```python
from build123d import *

# Parameters (mm, degrees)
F0_W        = 25
F0_H        = 25
F0_R        = 7.5
F1_DEPTH    = 35
F2_DEPTH    = 15
F3_SIZE2    = 21.650625
F3_SIZE     = 12.49999
F4_R        = 7.5
F5_DEPTH    = 5
F6_T1_DEPTH = 95.1228407313
F6_T3_DEPTH = 95.1228407313


# Not quite as in the source:
# - a fillet or chamfer that OpenCascade refuses, or shapes differently, is made with other operations: its cross-section is extruded or revolved along the edge and cut away or added
# - a fillet or chamfer is up to 0.001 mm smaller than in the source, because OpenCascade refuses the exact size


with BuildPart() as f1:
    # F0 (on Top) → F1 (new body)
    with BuildSketch(Plane.XY):
        with Locations((-12.5, -12.5)):
            Rectangle(F0_W, F0_H)
        with Locations((-12.5, -12.5)):
            Circle(F0_R, mode=Mode.SUBTRACT)
        with Locations((-12.5, -12.5)):
            Circle(F0_R)
    extrude(amount=F1_DEPTH)

    # F0 (on Top) → F2 (cut)
    with BuildSketch(Plane.XY):
        with Locations((-12.5, -12.5)):
            Circle(F0_R)
    extrude(amount=F2_DEPTH, mode=Mode.SUBTRACT)

    # F3 (size 12.5 and 21.6506350946 in the source; OpenCascade refuses exactly that, so slightly less here)
    f3_edges = [f1.edges().sort_by_distance(p)[0] for p in [
        (-25, -12.5, 35),
        (-12.5, -25, 35),
        (0, -12.5, 35),
        (-12.5, 0, 35),
    ]]
    f3_side = f1.faces().sort_by_distance((-12.5, -12.5, 35))[0]
    chamfer(f3_edges, length=F3_SIZE, length2=F3_SIZE2, reference=f3_side)

    # F4 (on Top) → F5 (join)
    with BuildSketch(Plane.XY):
        Polygon((-3.4594764784, -16.2579490188), (-3.4594764784, -8.802104896), (-8.731554417, -3.5300269574), (-16.1873985398, -3.5300269574), (-21.4594764784, -8.802104896), (-21.4594764784, -16.2579490188), (-16.1873985398, -21.5300269574), (-8.731554417, -21.5300269574), align=None)
        with Locations((-12.4594764784, -12.5300269574)):
            Circle(F4_R, mode=Mode.SUBTRACT)
    extrude(amount=-F5_DEPTH)

    # F6: chamfer of 13.5 x 3.3659280384 on 4 edges, made by hand

    # F6_s2 → F6_t1 (cut)
    with BuildSketch(Plane.YZ.offset(-60.0614203657)):
        Polygon((-25, 13.5), (-21.6340719616, 0), (-25, 0), align=None)
        Polygon((-3.3659280384, 0), (0, 13.5), (0, 0), align=None)
    extrude(amount=F6_T1_DEPTH, mode=Mode.SUBTRACT)

    # F6_s4 → F6_t3 (cut)
    with BuildSketch(Plane.XZ.offset(-35.0614203657)):
        Polygon((0, 13.5), (-3.3659280384, 0), (0, 0), align=None)
        Polygon((-21.6340719616, 0), (-25, 13.5), (-25, 0), align=None)
    extrude(amount=F6_T3_DEPTH, mode=Mode.SUBTRACT)


solid = f1.part
```
Verification items for the finished model (mm, model axes). A direction names the side the tool comes from. Coordinates: 2 decimals unless noted, no trailing zeros. Order: outer loops, then holes, each group sorted by start corner. A loop starts at its lowest first (then second) coordinate and runs counter-clockwise, first axis right, second up. Notation, with made-up numbers: (40.5, 6) -> (52.5, 6) arc R15 cw to (52.5, 27) -> close; hole circle Ø5 at (-9.75, -17). An arc over 180 degrees is marked (long way). Put each result on its own line as item: value. Start each with the question number.
1) Tool access check on faces 4 (the flat face through (-13, -21.53, -2)), 5 (the cylindrical face through (-14.13, -19.82, 7.4)), 6 (the cylindrical face through (-13.436, -5.094, -2.465)), 7 (the flat face through (-6.06, -6.2, -2.46)), 8 (the flat face through (-21.459, -12, -2)). Record the directions out of +Z, -Z, +X, -X, +Y, -Y that give a thin tool (end or side, any length) a straight path to the whole face; none if there is none.
2) Material ranges on L1, parallel to X at y = -12.5, z = 4.75; L2, parallel to X at y = -13.75, z = -1.5; L3, parallel to Y at x = -12.5, z = 3.25, recorded low to high.
3) Cross-section at D-D (y = -4). Enter the section's corners in (x, z).
4) Cross-section at C-C (z = 32). Enter the section's corners in (x, y), plus the area to 3 significant figures.
5) Go/stop test with flat-tipped pins: pin 1 (3 mm diameter, centred on x = -5, z = 25.5, fed in from -Y); pin 2 (5.5 mm diameter, centred on x = -12, z = -1.5, fed in from +Y); pin 3 (5 mm diameter, centred on y = -16, z = 17.5, fed in from +X); pin 4 (5.5 mm diameter, centred on y = -11, z = -3, fed in from -X). Record where each tip stops, or that it passes through.
6) Release check for a two-part mould opening along Y. For faces 1 (the flat face through (-13, -12, 15)), 2 (the flat face through (-6.1, -18.9, -2.5)), 3 (the flat face through (-3.459, -13, -2)) record: pulls with the +Y half, pulls with the -Y half, needs draft (parallel to the pull), parting line crosses it, or undercut.
Geometry check:
1. face 4: -Z, +X, -X, -Y
1. face 5: none
1. face 6: -Z
1. face 7: -Z, +X, +Y
1. face 8: -Z, -X, +Y, -Y
2. L1: x = -22.82 to -20, -5 to -2.18
2. L2: x = -21.46 to -19.86, -5.06 to -3.46
2. L3: y = -22.44 to -20, -5 to -2.56
3. outline: (-24.97, 13.39) -> (-21.63, 0) -> (-16.66, 0) -> (-16.66, -5) -> (-8.26, -5) -> (-8.26, 0) -> (-3.37, 0) -> (-0.03, 13.39) -> (-4, 20.28) -> (-21, 20.28) -> close
4. outline: (-14.23, -14.23) -> (-10.77, -14.23) -> (-10.77, -10.77) -> (-14.23, -10.77) -> close
4. area: 12.0 mm^2
5. pin 1: passes through
5. pin 2: stops at y = -3.05
5. pin 3: stops at x = -0.95
5. pin 4: stops at x = -21.46
6. face 1: undercut
6. face 2: pulls with the -Y half
6. face 3: needs draft
